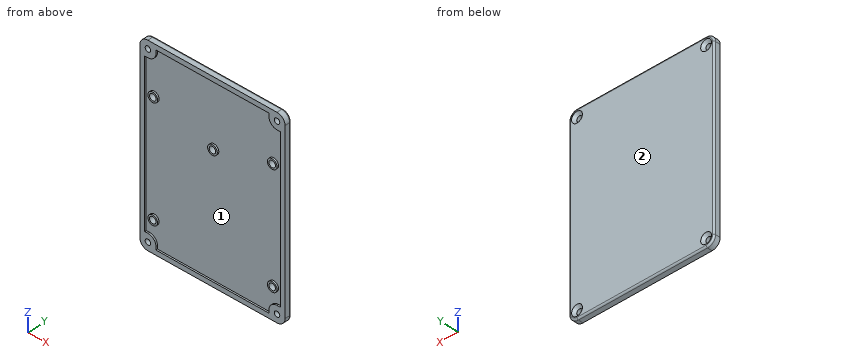
from build123d import *

# Parameters (mm, degrees)
SKETCH_2_W                  = 90
SKETCH_2_H                  = 120
EXTRUDE_1_DEPTH             = 3
SKETCH_3_W                  = 90
SKETCH_3_H                  = 120
EXTRUDE_2_DEPTH             = 1
HOLE_WIZARD_M3_3_AT_2_COUNT = 2
HOLE_WIZARD_M3_3_AT_2_PITCH = 110
HOLE_WIZARD_M3_3_AT_3_COUNT = 2
HOLE_WIZARD_M3_3_AT_3_PITCH = 136.014705087
HOLE_WIZARD_M3_3_AT_4_COUNT = 2
HOLE_WIZARD_M3_3_AT_4_PITCH = 80
FILLET_2_R                  = 5
FILLET_3_R                  = 5
FILLET_4_R                  = 5
FILLET_5_R                  = 5
FILLET_6_R                  = 5
FILLET_7_R                  = 5
FILLET_8_R                  = 5
FILLET_9_R                  = 5
FILLET_11_R                 = 1
SKETCH_18_R                 = 3
EXTRUDE_5_DEPTH             = 1
SKETCH_19_R                 = 2
CUT_EXTRUDE_1_DEPTH         = 3.1


with BuildPart() as part:
    # 草图2 → 凸台-拉伸1 (new body)
    with BuildSketch(Plane(origin=(0, 0, 0), x_dir=(1, 0, 0), z_dir=(0, 1, 0))):
        Rectangle(SKETCH_2_W, SKETCH_2_H)
    extrude(amount=EXTRUDE_1_DEPTH)


with BuildPart() as body_2:
    # 草图3 → 凸台-拉伸2 (new body)
    with BuildSketch(Plane.XZ):
        Rectangle(SKETCH_3_W, SKETCH_3_H)
        Polygon((-42, -50), (-42, 50), (-35, 50), (-35, 57), (35, 57), (35, 50), (42, 50), (42, -50), (35, -50), (35, -57), (-35, -57), (-35, -50), align=None, mode=Mode.SUBTRACT)
    extrude(amount=EXTRUDE_2_DEPTH)


with BuildPart() as hole_wizard_m3_3_tool:
    # 草图15 → M3 六角凹锥坑螺钉的锥形沉头孔3 (revolve)
    with BuildSketch(Plane(origin=(-40, 3, 55), x_dir=(0, 0, 1), z_dir=(1, 0, 0))):
        Polygon((0, 0), (0, 4), (1.7, 4), (1.7, 1.66), (3.36, 0), align=None)
    hole_wizard_m3_3 = revolve(axis=Axis((-40, 9.35, 55), (0, -1, 0)))


with BuildPart() as part_1:
    add(part.part)

    # M3 六角凹锥坑螺钉的锥形沉头孔3: cut by hole_wizard_m3_3_tool
    add(hole_wizard_m3_3_tool.part, mode=Mode.SUBTRACT)


with BuildPart() as body_2_1:
    add(body_2.part)

    # M3 六角凹锥坑螺钉的锥形沉头孔3: cut by hole_wizard_m3_3_tool
    add(hole_wizard_m3_3_tool.part, mode=Mode.SUBTRACT)


with BuildPart() as hole_wizard_m3_3_at_2_tool:
    # M3 六角凹锥坑螺钉的锥形沉头孔3 at 2: M3 六角凹锥坑螺钉的锥形沉头孔3 ×2
    with Locations(*[(0, 0, -i * HOLE_WIZARD_M3_3_AT_2_PITCH) for i in range(1, HOLE_WIZARD_M3_3_AT_2_COUNT)]):
        add(hole_wizard_m3_3)


with BuildPart() as part_2:
    add(part_1.part)

    # M3 六角凹锥坑螺钉的锥形沉头孔3 at 2: cut by hole_wizard_m3_3_at_2_tool
    add(hole_wizard_m3_3_at_2_tool.part, mode=Mode.SUBTRACT)


with BuildPart() as body_2_2:
    add(body_2_1.part)

    # M3 六角凹锥坑螺钉的锥形沉头孔3 at 2: cut by hole_wizard_m3_3_at_2_tool
    add(hole_wizard_m3_3_at_2_tool.part, mode=Mode.SUBTRACT)


with BuildPart() as hole_wizard_m3_3_at_3_tool:
    # M3 六角凹锥坑螺钉的锥形沉头孔3 at 3: M3 六角凹锥坑螺钉的锥形沉头孔3 ×2
    with Locations(*[Vector(0.5881716976750462, 0, -0.8087360843031886) * (i * HOLE_WIZARD_M3_3_AT_3_PITCH) for i in range(1, HOLE_WIZARD_M3_3_AT_3_COUNT)]):
        add(hole_wizard_m3_3)


with BuildPart() as part_3:
    add(part_2.part)

    # M3 六角凹锥坑螺钉的锥形沉头孔3 at 3: cut by hole_wizard_m3_3_at_3_tool
    add(hole_wizard_m3_3_at_3_tool.part, mode=Mode.SUBTRACT)


with BuildPart() as body_2_3:
    add(body_2_2.part)

    # M3 六角凹锥坑螺钉的锥形沉头孔3 at 3: cut by hole_wizard_m3_3_at_3_tool
    add(hole_wizard_m3_3_at_3_tool.part, mode=Mode.SUBTRACT)


with BuildPart() as hole_wizard_m3_3_at_4_tool:
    # M3 六角凹锥坑螺钉的锥形沉头孔3 at 4: M3 六角凹锥坑螺钉的锥形沉头孔3 ×2
    with Locations(*[(i * HOLE_WIZARD_M3_3_AT_4_PITCH, 0, 0) for i in range(1, HOLE_WIZARD_M3_3_AT_4_COUNT)]):
        add(hole_wizard_m3_3)


with BuildPart() as part_4:
    add(part_3.part)

    # M3 六角凹锥坑螺钉的锥形沉头孔3 at 4: cut by hole_wizard_m3_3_at_4_tool
    add(hole_wizard_m3_3_at_4_tool.part, mode=Mode.SUBTRACT)


with BuildPart() as body_2_4:
    add(body_2_3.part)

    # M3 六角凹锥坑螺钉的锥形沉头孔3 at 4: cut by hole_wizard_m3_3_at_4_tool
    add(hole_wizard_m3_3_at_4_tool.part, mode=Mode.SUBTRACT)

    # Combine 2: union part
    add(part_4.part)

    # 圆角2
    fillet_2_edges = [body_2_4.edges().sort_by_distance(p)[0] for p in [
        (35, -0.5, -50),
    ]]
    fillet(fillet_2_edges, radius=FILLET_2_R)

    # 圆角3
    fillet_3_edges = [body_2_4.edges().sort_by_distance(p)[0] for p in [
        (-35, -0.5, -50),
    ]]
    fillet(fillet_3_edges, radius=FILLET_3_R)

    # 圆角4
    fillet_4_edges = [body_2_4.edges().sort_by_distance(p)[0] for p in [
        (35, -0.5, 50),
    ]]
    fillet(fillet_4_edges, radius=FILLET_4_R)

    # 圆角5
    fillet_5_edges = [body_2_4.edges().sort_by_distance(p)[0] for p in [
        (-35, -0.5, 50),
    ]]
    fillet(fillet_5_edges, radius=FILLET_5_R)

    # 圆角6
    fillet_6_edges = [body_2_4.edges().sort_by_distance(p)[0] for p in [
        (-45, 1, -60),
    ]]
    fillet(fillet_6_edges, radius=FILLET_6_R)

    # 圆角7
    fillet_7_edges = [body_2_4.edges().sort_by_distance(p)[0] for p in [
        (45, 1, -60),
    ]]
    fillet(fillet_7_edges, radius=FILLET_7_R)

    # 圆角8
    fillet_8_edges = [body_2_4.edges().sort_by_distance(p)[0] for p in [
        (45, 1, 60),
    ]]
    fillet(fillet_8_edges, radius=FILLET_8_R)

    # 圆角9
    fillet_9_edges = [body_2_4.edges().sort_by_distance(p)[0] for p in [
        (-45, 1, 60),
    ]]
    fillet(fillet_9_edges, radius=FILLET_9_R)

    # 圆角11
    fillet_11_edges = [body_2_4.edges().sort_by_distance(p)[0] for p in [
        (-45, 3, 0),
        (-43.535533906, 3, -58.535533906),
        (0, 3, -60),
        (43.535533906, 3, -58.535533906),
        (45, 3, 0),
        (43.535533906, 3, 58.535533906),
        (0, 3, 60),
        (-43.535533906, 3, 58.535533906),
    ]]
    fillet(fillet_11_edges, radius=FILLET_11_R)

    # 草图18 → 凸台-拉伸5 (add)
    with BuildSketch(Plane.XZ):
        with Locations(Location((-37, 29, 0), (0, 0, 90))):
            Circle(SKETCH_18_R)
        with Locations(Location((37, 29, 0), (0, 0, 90))):
            Circle(SKETCH_18_R)
        with Locations(Location((0, 18, 0), (0, 0, 90))):
            Circle(SKETCH_18_R)
        with Locations(Location((-37, -41, 0), (0, 0, 90))):
            Circle(SKETCH_18_R)
        with Locations(Location((37, -41, 0), (0, 0, 90))):
            Circle(SKETCH_18_R)
    extrude(amount=EXTRUDE_5_DEPTH)

    # 草图19 → 切除-拉伸1 (cut)
    with BuildSketch(Plane.XZ.offset(1)):
        with Locations(Location((-37, 29, 0), (0, 0, 270))):
            Circle(SKETCH_19_R)
        with Locations(Location((37, 29, 0), (0, 0, 270))):
            Circle(SKETCH_19_R)
        with Locations(Location((0, 18, 0), (0, 0, 270))):
            Circle(SKETCH_19_R)
        with Locations(Location((-37, -41, 0), (0, 0, 270))):
            Circle(SKETCH_19_R)
        with Locations(Location((37, -41, 0), (0, 0, 270))):
            Circle(SKETCH_19_R)
    extrude(amount=-CUT_EXTRUDE_1_DEPTH, mode=Mode.SUBTRACT)


solid = body_2_4.part
Check sheet for the modelled part. Datum: model origin and axes. Units: mm. Face numbers are marked on the shaded views. Give positions to 0.01 mm unless a question says otherwise; leave off trailing zeros. Order: outer loops, then holes, each group sorted by start corner. A loop starts at its lowest first (then second) coordinate and runs counter-clockwise, first axis right, second up. Notation, with made-up numbers: (46, 80.5) - (68, 80.5) arc R22 cw to (68, 118.5) - close; hole circle Ø4 at (-4.75, 88.5). An arc over 180 degrees is marked (long way). Answer as CSV lines item,"result".
1. Mould release check, pull along Z, two halves, no side actions. Record for the marked faces 1 and 2: released by +Z, released by -Z, zero draft, split by the parting line, or undercut.
Result sheet:
face 1,"undercut"
face 2,"zero draft"
2. Section check B-B (z = 18). Record the boundary of the cut face in (x, y).
Result sheet:
outline,"(-45, -1) - (-42, -1) - (-42, 0) - (-3, 0) - (-3, -1) - (-2, -1) - (-2, 2.1) - (2, 2.1) - (2, -1) - (3, -1) - (3, 0) - (42, 0) - (42, -1) - (45, -1) - (45, 2) arc R1 ccw to (44, 3) - (-44, 3) arc R1 ccw to (-45, 2) - close"
3. Section check A-A (x = 11.5). Record the boundary of the cut face in (y, z), then the cut area to 3 significant figures.
Result sheet:
outline,"(-1, -60) - (2, -60) arc R1 ccw to (3, -59) - (3, 59) arc R1 ccw to (2, 60) - (-1, 60) - (-1, 57) - (0, 57) - (0, -57) - (-1, -57) - close"
area,"366 mm²"
4. Go/stop test with flat-tipped pins: P1, Ø1.1, axis at y = -0.5, z = -56.5, coming from the -X side; P2, Ø2.5, axis at x = 40, z = 55, coming from the +Y side; P3, Ø2.5, axis at x = -37, z = -41, coming from the -Y side; P4, Ø4.5, axis at x = -40, z = 55, coming from the +Y side. Record where each tip stops, or that it passes through.
Result sheet:
P1,"x = -44.91"
P2,"through"
P3,"y = 2.1"
P4,"y = 1.89"
5. Section check C-C (z = 1). Record the boundary of the cut face in (x, y).
Result sheet:
outline,"(-45, -1) - (-42, -1) - (-42, 0) - (42, 0) - (42, -1) - (45, -1) - (45, 2) arc R1 ccw to (44, 3) - (-44, 3) arc R1 ccw to (-45, 2) - close"
6. Scan lines: probe 1 along Z at (x, y) = (40, 0.85); probe 2 along X at (y, z) = (0.2, 29); probe 3 along X at (y, z) = (-0.1, -41). Record each from-to range of solid material in increasing order. Write a range as from..to.
Result sheet:
probe 1,"-60..-56.7, -53.3..53.3, 56.7..60"
probe 2,"-45..-39, -35..35, 39..45"
probe 3,"-45..-42, -40..-39, -35..-34, 34..35, 39..40, 42..45"
